Here's how the part is built. I have some questions about the finished solid (model axes, mm). A direction names the side the tool comes from. Coordinates: 2 decimals unless noted, no trailing zeros. Write each loop counter-clockwise with the first axis right and the second up, starting at its lowest first coordinate (ties: lowest second). Pieces come first, ordered by that corner, then holes. Notation, with made-up numbers: (-33, 78) -> (-28, 78) arc R14 cw to (-28, 93) -> close; hole circle Ø11 at (59, -1.5). An arc over 180 degrees is marked (long way). Use a Markdown table: item, result. Add a question column.
Item 1: Imagine slicing it at A-A, the plane z = 0. Write out the boundary of the cut face in (x, y).
Item 2: Imagine slicing it at B-B, the plane x = 0. Write out the boundary of the cut face in (y, z), and give its area (3 significant figures).
Item 3: Imagine slicing it at C-C, the plane y = 192.5. Write out the boundary of the cut face in (x, z), and give its area (3 significant figures).
Item 4: On a 3-axis mill with a long thin cutter (end or side, diameter ignored), from which of +Z, -Z, +X, -X, +Y, -Y can I reach the whole of each face in a straight line? I mean faces 5 (the flat face through (0, 184, 6)), 6 (the flat face through (0, 184, -6)), 7 (the flat face through (-9, 183, 0)), 8 (the cylindrical face through (0, 84, 5)). Say none if no direction works.
Item 5: Will these pins go through, and if not, where does the flat tip stop? pin 1 Ø6 at (y, z) = (191.5, -2.5) entering from +X; pin 2 Ø10 at (y, z) = (102.5, -5.5) entering from +X; pin 3 Ø9.5 at (y, z) = (176, -1.5) entering from -X.
Item 6: If we mould it in two halves opening along Y, with no side actions, what happens to faces 1 (the flat face through (0, -20, 0)), 2 (the cylindrical face through (-0.651, 197.457, -0.084)), 3 (the flat face through (9, 183, 0)), 4 (the flat face through (-5, 0, -2))? For each: pulls with the +Y half, pulls with the -Y half, needs draft (parallel to the pull), parting line crosses it, or undercut.
Item 7: If I drill on line 1 along Y through (x, z) = (0, -1.5); line 2 along Z through (x, y) = (7, 175.5); line 3 along Y through (x, z) = (0.25, 8.5), over which ranges is the centre line in solid material (lowest first)? Write a range as from..to.
Item 8: Imagine slicing it at D-D, the plane y = 4.5. Write out the boundary of the cut face in (x, z).
```python
from build123d import *

# Parameters (mm, degrees)
ESQUISSE1_W        = 5
ESQUISSE1_H        = 165
ESQUISSE2_W        = 10
ESQUISSE2_H        = 20
ESQUISSE3_W        = 18
ESQUISSE3_H        = 36.5
ESQUISSE3_R        = 5
BOSS_EXTRU_1_DEPTH = 6


with BuildPart() as part:
    # Esquisse1 → Base-Révolution (revolve)
    with BuildSketch(Plane.XY, mode=Mode.PRIVATE) as base_r_volution_sk:
        with Locations((2.5, 82.5)):
            Rectangle(ESQUISSE1_W, ESQUISSE1_H)
    revolve(base_r_volution_sk.sketch.rotate(Axis((0, -40, 0), (0, 1, 0)), 90), axis=Axis((0, -40, 0), (0, 1, 0)))

    # Esquisse2 → Boss.-Révol.1 (revolve)
    with BuildSketch(Plane.XY, mode=Mode.PRIVATE) as boss_r_vol_1_sk:
        with Locations((5, -10)):
            Rectangle(ESQUISSE2_W, ESQUISSE2_H)
    revolve(boss_r_vol_1_sk.sketch.rotate(Axis((0, 0, 0), (0, -1, 0)), 90), axis=Axis((0, 0, 0), (0, -1, 0)))

    # Esquisse3 → Boss.-Extru.1 (add, symmetric)
    with BuildSketch(Plane.XY):
        with Locations((0, 183.25)):
            Rectangle(ESQUISSE3_W, ESQUISSE3_H)
        with Locations((0, 192.5)):
            Circle(ESQUISSE3_R, mode=Mode.SUBTRACT)
    extrude(amount=BOSS_EXTRU_1_DEPTH, both=True)


solid = part.part
```
Ans:
| question | item | result |
|---|---|---|
| 1 | outline | (-10, -20) -> (10, -20) -> (10, 0) -> (5, 0) -> (5, 165) -> (9, 165) -> (9, 201.5) -> (-9, 201.5) -> (-9, 165) -> (-5, 165) -> (-5, 0) -> (-10, 0) -> close; hole circle Ø10 at (0, 192.5) |
| 2 | outline | (-20, -10) -> (0, -10) -> (0, -5) -> (165, -5) -> (165, -6) -> (187.5, -6) -> (187.5, 6) -> (165, 6) -> (165, 5) -> (0, 5) -> (0, 10) -> (-20, 10) -> close; (197.5, -6) -> (201.5, -6) -> (201.5, 6) -> (197.5, 6) -> close |
| 2 | area | 2,370 mm^2 |
| 3 | outline | (-9, -6) -> (-5, -6) -> (-5, 6) -> (-9, 6) -> close; (5, -6) -> (9, -6) -> (9, 6) -> (5, 6) -> close |
| 3 | area | 96.0 mm^2 |
| 4 | face 5 | +Z, +X, -X, +Y |
| 4 | face 6 | -Z, +X, -X, +Y |
| 4 | face 7 | +Z, -Z, -X, +Y |
| 4 | face 8 | none |
| 5 | pin 1 | stops at x = 9 |
| 5 | pin 2 | stops at x = 4.97 |
| 5 | pin 3 | stops at x = -9 |
| 6 | face 1 | pulls with the -Y half |
| 6 | face 2 | undercut |
| 6 | face 3 | needs draft |
| 6 | face 4 | undercut |
| 7 | line 1 | y = -20..187.5, 197.5..201.5 |
| 7 | line 2 | z = -6..6 |
| 7 | line 3 | y = -20..0 |
| 8 | outline | circle Ø10 at (0, 0) |
